Input: part model. Units: mm. Frame: model coordinates. A direction names the side the tool comes from. Round coordinates to 2 decimals unless told otherwise and drop trailing zeros. Write each loop counter-clockwise with the first axis right and the second up, starting at its lowest first coordinate (ties: lowest second). Pieces come first, ordered by that corner, then holes. Notation, with made-up numbers: (73, 75.25) -> (130, 75.25) arc R24 ccw to (130, 103.25) -> close; hole circle Ø10 at (48.5, -14). An arc over 180 degrees is marked (long way). Use CSV: the item, a comma, the result in double quotes.
```python
from build123d import *

# Parameters (mm, degrees)
SKETCH1_R           = 14.5
SKETCH1_R_2         = 9.85
BOSS_EXTRUDE1_DEPTH = 9
SKETCH2_R           = 14.5
SKETCH2_R_2         = 12.5
BOSS_EXTRUDE2_DEPTH = 37.5


with BuildPart() as part:
    # Sketch1 → Boss-Extrude1 (new body, symmetric)
    with BuildSketch(Plane.XY):
        Circle(SKETCH1_R)
        Circle(SKETCH1_R_2, mode=Mode.SUBTRACT)
    extrude(amount=BOSS_EXTRUDE1_DEPTH, both=True)

    # Sketch2 → Boss-Extrude2 (add, symmetric)
    with BuildSketch(Plane.XY):
        Circle(SKETCH2_R)
        Circle(SKETCH2_R_2, mode=Mode.SUBTRACT)
    extrude(amount=BOSS_EXTRUDE2_DEPTH, both=True)


solid = part.part
```
Item 1: Set-up query: faces 1 (the face through (-9.32, -3.65, -9)), 2 (the face through (-7.82, -5.99, -0.13)). Return all of +Z, -Z, +X, -X, +Y, -Y with unobstructed straight access to the full face (end or side cutting, diameter ignored); none if empty.
Worked answers:
face 1,"-Z"
face 2,"+Z, -Z"
Item 2: Line query: line 1 (Y direction, x = 0, z = 1.25); line 2 (Y direction, x = 0, z = 18); line 3 (Z direction, x = -11.75, y = 0.25). Output: solid intervals per line, ascending.
Worked answers:
line 1,"y = -14.5 to -9.85, 9.85 to 14.5"
line 2,"y = -14.5 to -12.5, 12.5 to 14.5"
line 3,"z = -9 to 9"
Item 3: Section query A-A on x = 0. Return the cut outline in (y, z), plus the area to 3 significant figures.
Worked answers:
outline,"(-14.5, -37.5) -> (-12.5, -37.5) -> (-12.5, -9) -> (-9.85, -9) -> (-9.85, 9) -> (-12.5, 9) -> (-12.5, 37.5) -> (-14.5, 37.5) -> close; (9.85, -9) -> (12.5, -9) -> (12.5, -37.5) -> (14.5, -37.5) -> (14.5, 37.5) -> (12.5, 37.5) -> (12.5, 9) -> (9.85, 9) -> close"
area,"395 mm²"
Item 4: Section query C-C on z = -17. Return the cut outline in (x, y), plus the area to 3 significant figures.
Worked answers:
outline,"circle Ø29 at (0, 0); hole circle Ø25 at (0, 0)"
area,"170 mm²"
Item 5: First-contact query: pin 1 Ø8 at (x, z) = (-10, -14.5) entering from -Y; pin 2 Ø12.5 at (x, y) = (1, 1) entering from -Z; pin 3 Ø8 at (x, y) = (-6.5, -4.5) entering from -Z; pin 4 Ø12.5 at (x, y) = (6, 1.5) entering from +Z. Flat tips, straight axial feed; report the tip coordinate or a pass-through.
Worked answers:
pin 1,"stops at y = -13.2"
pin 2,"passes through"
pin 3,"stops at z = -9"
pin 4,"stops at z = 9"
Item 6: Pull-direction query (X, two-part tool) for faces 3 (the face through (6.691, -12.864, 0.525)), 4 (the face through (-9.32, -3.65, 9)), 5 (the face through (11.923, 3.755, 23.05)), 6 (the face through (-11, 7, 37.5)); classes: +X half, -X half, draft (parallel to the pull), parting line (faces both ways), or undercut.
Worked answers:
face 3,"parting line"
face 4,"undercut"
face 5,"undercut"
face 6,"draft"
Item 7: Section query D-D on z = 5. Return the cut outline in (x, y), plus the area to 3 significant figures.
Worked answers:
outline,"circle Ø29 at (0, 0); hole circle Ø19.7 at (0, 0)"
area,"356 mm²"
